Input: part model. Units: mm. Frame: model coordinates. Face numbers are marked on the shaded views. Give positions to 0.01 mm unless a question says otherwise; leave off trailing zeros. Order: outer loops, then holes, each group sorted by start corner. A loop starts at its lowest first (then second) coordinate and runs counter-clockwise, first axis right, second up. Notation, with made-up numbers: M -0.75,-32.75 L 39.25,-32.75 A25 cw 39.25,-9.75 Z; hole C 57,43 d3. An arc over 180 degrees is marked long. Use a Markdown table: item, result.
from build123d import *
from OCP.BRepFilletAPI import BRepFilletAPI_MakeChamfer

# Parameters (mm, degrees)
SKETCH1_R           = 1.6
BOSS_EXTRUDE1_DEPTH = 3
SKETCH3_W           = 31.2
SKETCH3_H           = 3
BOSS_EXTRUDE2_DEPTH = 60
BOSS_EXTRUDE3_DEPTH = 60
CHAMFER1_SIZE       = 5
CHAMFER1_SIZE2      = 3.535533906
CHAMFER2_SIZE       = 2
CHAMFER3_SIZE       = 2
CHAMFER4_SIZE       = 2
SKETCH5_W           = 12.1
SKETCH5_H           = 20.1
CUT_EXTRUDE1_DEPTH  = 30
SKETCH6_R           = 4.75
CUT_EXTRUDE2_DEPTH  = 30
CHAMFER5_SIZE       = 10


with BuildPart() as part:
    # Sketch1 → Boss-Extrude1 (new body)
    with BuildSketch(Plane.XY):
        with BuildLine():
            ThreePointArc((-11, 4.6), (-14.252691193, 3.252691193), (-15.6, 0))
            Line((-15.6, 0), (-15.6, -25))
            Line((-15.6, -25), (15.6, -25))
            Line((15.6, -25), (15.6, 0))
            ThreePointArc((15.6, 0), (14.252691193, 3.252691193), (11, 4.6))
            Line((11, 4.6), (-11, 4.6))
        make_face()
        with Locations((-11, 0)):
            Circle(SKETCH1_R, mode=Mode.SUBTRACT)
        with Locations((11, 0)):
            Circle(SKETCH1_R, mode=Mode.SUBTRACT)
    extrude(amount=BOSS_EXTRUDE1_DEPTH)

    # Sketch3 → Boss-Extrude2 (add)
    with BuildSketch(Plane(origin=(0, 0, 0), x_dir=(-1, 0, 0), z_dir=(0, 0, -1))):
        with Locations((0, -26.5)):
            Rectangle(SKETCH3_W, SKETCH3_H)
    extrude(amount=-BOSS_EXTRUDE2_DEPTH)

    # Sketch4 → Boss-Extrude3 (add)
    with BuildSketch(Plane(origin=(0, 0, 0), x_dir=(-1, 0, 0), z_dir=(0, 0, -1))):
        Polygon((-15.6, -28), (-15.6, -20.928932188), (-22.671067812, -28), align=None)
        Polygon((15.6, -20.928932188), (15.6, -28), (22.671067812, -28), align=None)
    extrude(amount=-BOSS_EXTRUDE3_DEPTH)

    # Chamfer1: one chamfer whose edges measure the first distance from different faces: ONE call of the kernel's chamfer builder (chamfer() names one face for all edges)
    chamfer1_edges_1 = [part.edges().sort_by_distance(p)[0] for p in [
        (0, -28, 0),
    ]]
    chamfer1_edges_2 = [part.edges().sort_by_distance(p)[0] for p in [
        (22.671067812, -28, 30),
    ]]
    chamfer1_side_2 = [part.faces().sort_by_distance(p)[0] for p in [
        (0, -28, 30),
    ]]
    chamfer1_edges_3 = [part.edges().sort_by_distance(p)[0] for p in [
        (-22.671067812, -28, 30),
    ]]
    chamfer1_side_3 = [part.faces().sort_by_distance(p)[0] for p in [
        (-19.135533906, -24.464466094, 30),
    ]]
    chamfer1 = BRepFilletAPI_MakeChamfer(part.part.solid().wrapped)
    for e in chamfer1_edges_1:
        chamfer1.Add(CHAMFER1_SIZE, e.wrapped)
    for e in chamfer1_edges_2:
        chamfer1.Add(CHAMFER1_SIZE, CHAMFER1_SIZE2, e.wrapped, chamfer1_side_2[0].wrapped)  # the first distance lies on this face
    for e in chamfer1_edges_3:
        chamfer1.Add(CHAMFER1_SIZE, CHAMFER1_SIZE2, e.wrapped, chamfer1_side_3[0].wrapped)  # the first distance lies on this face
    add(Compound.cast(chamfer1.Shape()), mode=Mode.REPLACE)

    # Chamfer2
    chamfer2_edges = [part.edges().sort_by_distance(p)[0] for p in [
        (14.252691193, 3.252691193, 0),
        (15.6, -10.464466094, 0),
        (-15.6, -10.464466094, 0),
        (-14.252691193, 3.252691193, 0),
        (0, 4.6, 0),
    ]]
    chamfer(chamfer2_edges, length=CHAMFER2_SIZE)

    # Chamfer3
    chamfer3_edges = [part.edges().sort_by_distance(p)[0] for p in [
        (-19.135533906, -28, 32.5),
    ]]
    chamfer(chamfer3_edges, length=CHAMFER3_SIZE)

    # Chamfer4
    chamfer4_edges = [part.edges().sort_by_distance(p)[0] for p in [
        (20.171067812, -25.5, 31.25),
    ]]
    chamfer(chamfer4_edges, length=CHAMFER4_SIZE)

    # Sketch5 → Cut-Extrude1 (cut)
    with BuildSketch(Plane.XZ.offset(28)):
        with Locations((0.267766953, 35.55312029)):
            Rectangle(SKETCH5_W, SKETCH5_H)
    extrude(amount=-CUT_EXTRUDE1_DEPTH, mode=Mode.SUBTRACT)

    # Sketch6 → Cut-Extrude2 (cut)
    with BuildSketch(Plane.XZ.offset(28)):
        with Locations((9.761183066, 14.413738274)):
            Circle(SKETCH6_R)
        with Locations(Location((-9.761183066, 14.413738274, 0), (0, 0, 270))):
            Circle(SKETCH6_R)
    extrude(amount=-CUT_EXTRUDE2_DEPTH, mode=Mode.SUBTRACT)

    # Chamfer5
    # the kernel refuses this chamfer: 10 mm, written as the material it takes off along each edge
    with BuildSketch(Plane(origin=(-37.320078704, -7.815455201, 60), x_dir=(-0.019442520806014, -0.01944252080601393, -0.9996219169112968), z_dir=(0.7071067811865462, -0.7071067811865488, 0))) as chamfer5_piece_1:
        Polygon((CHAMFER5_SIZE * 0.999621916911, CHAMFER5_SIZE * 0.0274958766106), (-CHAMFER5_SIZE * 0.0274958766106, CHAMFER5_SIZE * 0.999621916911), (0, 0), align=None)
    extrude(amount=54.262086884, mode=Mode.SUBTRACT)
    with BuildSketch(Plane(origin=(-0.513476987, -46.184544799, 60), x_dir=(0.019442520806014572, -0.019442520806014493, -0.9996219169112968), z_dir=(0.7071067811865461, 0.707106781186549, 0))) as chamfer5_piece_2:
        Polygon((CHAMFER5_SIZE * 0.999621916911, CHAMFER5_SIZE * 0.0274958766106), (-CHAMFER5_SIZE * 0.0274958766106, CHAMFER5_SIZE * 0.999621916911), (0, 0), align=None)
    extrude(amount=52.969193665, mode=Mode.SUBTRACT)


solid = part.part
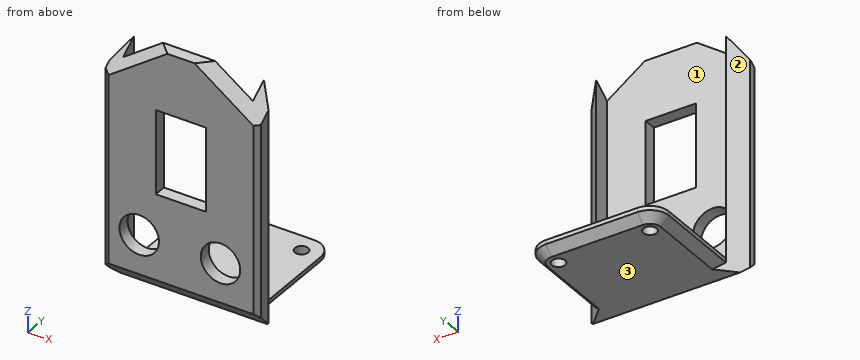
1) Cut plane B-B on y = -6. Return loops of the section in (x, z).
Response values:
| item | result |
|---|---|
| outline | M -15.6,2 L -13.6,0 L 13.6,0 L 15.6,2 L 15.6,3 L -15.6,3 Z |
2) Cut plane C-C on z = 55. Return loops of the section in (x, y), and give its area (3 significant figures).
Response values:
| item | result |
|---|---|
| outline | M -16.37,-21.7 L -15.6,-22.46 L -15.6,-20.93 Z; M -13.06,-25 L -10.06,-28 L 10.6,-28 L 13.6,-25 Z; M 15.6,-23 L 16.64,-21.96 L 15.6,-20.93 Z |
| area | 72.7 mm² |
3) Cut plane A-A on z = 34. Return loops of the section in (x, y).
Response values:
| item | result |
|---|---|
| outline | M -19.14,-26 L -17.14,-28 L -5.78,-28 L -5.78,-25 L -15.6,-25 L -15.6,-20.93 L -19.14,-24.46 Z; M 6.32,-28 L 17.67,-28 L 18.76,-26.91 L 18.76,-24.09 L 15.6,-20.93 L 15.6,-25 L 6.32,-25 Z |
4) First-contact query: pin 1 Ø1.5 at (x, y) = (-2.5, -26) entering from -Z; pin 2 Ø2 at (y, z) = (-22, 27.5) entering from -X; pin 3 Ø4 at (x, y) = (-3, -14) entering from -Z; pin 4 Ø5.5 at (x, z) = (9.76, 14.41) entering from +Y. Flat tips, straight axial feed; report the tip coordinate or a pass-through.
Response values:
| item | result |
|---|---|
| pin 1 | stops at z = 2.25 |
| pin 2 | stops at x = -17.67 |
| pin 3 | stops at z = 0 |
| pin 4 | passes through |
5) Mould query, pull axis X, two halves, no side actions, for the marked faces 1, 2 and 3. Classes: released by +X, released by -X, zero draft, split by the parting line, or undercut.
Response values:
| item | result |
|---|---|
| face 1 | undercut |
| face 2 | released by -X |
| face 3 | zero draft |
6) Material intervals for line 1 (X direction, y = -26, z = 39.5); line 2 (Y direction, x = -4, z = 15.5); line 3 (Z direction, x = -7, y = -22), sorted ascending. Write a range as from..to.
Response values:
| item | result |
|---|---|
| line 1 | x = -19.14..-5.78, 6.32..18.76 |
| line 2 | y = -28..-25 |
| line 3 | z = 0..3 |
